Geometry: final body of the model. Coordinates: model frame, mm. A direction names the side the tool comes from. Round coordinates to 2 decimals unless told otherwise and drop trailing zeros. Loops run counter-clockwise (first coordinate to the right, second up) from the corner with the lowest first, then second, coordinate; pieces in that order, holes last. Notation, with made-up numbers: (33.5, 15.25) - (65.5, 15.25) arc R24 ccw to (65.5, 51.25) - close; hole circle Ø2 at (-26.5, 8.5). An arc over 180 degrees is marked (long way). Answer as a JSON object with one key per item and string values. Group by question number.
Item 1: Section A-A (z = 0). Return the cut outline in (x, y).
Item 2: Line query: line 1 (Z direction, x = -14, y = 2.2); line 2 (X direction, y = 1.25, z = 0); line 3 (X direction, y = 1.7, z = 16). Output: solid intervals per line, ascending.
Item 3: Section C-C (y = 0.65). Return the cut outline in (x, z).
Item 4: Section B-B (x = 1). Return the cut outline in (y, z), plus the area to 3 significant figures.
Item 5: Draft query along Z for faces 1 (the face through (-2, 1, -9)), 2 (the face through (2.863, 1.479, 0.969)), 3 (the face through (-9.248, 1.521, 9.713)). Return one class per face: released by +Z, released by -Z, zero draft, split by the parting line, or undercut.
Item 6: Reachability of faces 4 (the face through (-17.4, 1.48, 19.43)), 5 (the face through (-10, 1, -15)), 6 (the face through (-10, 1, 15)) from +Z, -Z, +X, -X, +Y, -Y: full face, straight path, thin tool, end or side. Return the list, or none.
Item 7: Section D-D (x = -14). Return the cut outline in (y, z), plus the area to 3 significant figures.
Item 8: First-contact query: pin 1 (0.9 mm diameter, centred on y = 1.5, z = 16, fed in from +X); pin 2 (4 mm diameter, centred on x = 1, z = 0, fed in from -Y). Flat tips, straight axial feed; report the tip coordinate or a pass-through.
Autodesk Inventor part; units mm, degrees
ref_plane "YZ Plane" through (0, 0, 0) normal (1, 0, 0) x (0, 1, 0)
ref_plane "XZ Plane" through (0, 0, 0) normal (0, 1, 0) x (-1, 0, 0)
ref_plane "XY Plane" through (0, 0, 0) normal (0, 0, 1) x (1, 0, 0)
sketch "スケッチ1" plane through (0, 0, 0) normal (0, 1, 0) x (-1, 0, 0)
  line L0 (-3, 9) -> (10, 9)
  line L1 (10, -9) -> (-3, -9)
  line L2 (-5, -7) -> (-5, 7)
  line L3 (12, 20) -> (16, 20)
  line L4 (18, 18) -> (18, -18)
  line L5 (16, -20) -> (12, -20)
  line L6 (10, -18) -> (10, -9)
  line L7 (10, 9) -> (10, 18)
  arc A0 (18, 18) -> (16, 20) centre (16, 18) ccw
  arc A1 (12, 20) -> (10, 18) centre (12, 18) ccw
  arc A2 (16, -20) -> (18, -18) centre (16, -18) ccw
  arc A3 (10, -18) -> (12, -20) centre (12, -18) ccw
  arc A4 (-5, -7) -> (-3, -9) centre (-3, -7) ccw
  arc A5 (-3, 9) -> (-5, 7) centre (-3, 7) ccw
  point P0 (0, 0)
  point P1 (-5, 9)
  point P2 (-5, -9)
  point P3 (10, 20)
  point P4 (18, -20)
  point P5 (18, 20)
  point P6 (10, -20)
  dimension "d0" = 5
  dimension "d2" = 8
  dimension "d3" = 8
  dimension "d4" = 18
  dimension "d5" = 9
  dimension "d6" = 40
  dimension "d7" = 20
  dimension "d8" = 10
  dimension "d10" = 2
extrude "プレート1" add sketch "スケッチ1" along normal blind 3
hole "穴1" at (-14, 3, 16) direction (0, -1, 0) diameter 4.2 end through all
hole "穴2" at (-14, 3, -16) direction (0, -1, 0) diameter 4.2 end through all
hole "穴3" at (1, 3, 0) direction (0, -1, 0) diameter 4.2 end through all
sketch "スケッチ2" plane through (0, 0, 0) normal (0, -1, 0) x (1, 0, 0)
  circle A0 centre (1, 0) radius 2.1
  circle A1 centre (-14, -16) radius 2.1
  circle A2 centre (-14, 16) radius 2.1
  line L0 (-10, 9) -> (3, 9)
  line L1 (-10, 18) -> (-10, 9)
  arc A3 (-10, 18) -> (-12, 20) centre (-12, 18) ccw
  line L2 (-16, 20) -> (-12, 20)
  arc A4 (-16, 20) -> (-18, 18) centre (-16, 18) ccw
  line L3 (-18, -18) -> (-18, 18)
  arc A5 (-18, -18) -> (-16, -20) centre (-16, -18) ccw
  line L4 (-12, -20) -> (-16, -20)
  arc A6 (-12, -20) -> (-10, -18) centre (-12, -18) ccw
  line L5 (-10, -9) -> (-10, -18)
  line L6 (3, -9) -> (-10, -9)
  arc A7 (3, -9) -> (5, -7) centre (3, -7) ccw
  line L7 (5, 7) -> (5, -7)
  arc A8 (5, 7) -> (3, 9) centre (3, 7) ccw
  point P0 (0, 0)
fillet "フィレット1" radius 2.5 2 edges at (-10, 1.5, 9) (-10, 1.5, -9)
equation "\"d3\" = d2"
equation "\"d18\" = Thickness"
equation "\"d28\" = Thickness"
equation "\"d37\" = Thickness"
equation "\"d9\" = Thickness"
equation "\"BendRadius\" = Thickness"
equation "\"BendReliefWidth\" = Thickness"
equation "\"BendReliefDepth\" = 0.5 * Thickness"
equation "\"CornerReliefSize\" = 4 * Thickness"
equation "\"MinimumRemnant\" = 2 * Thickness"
equation "\"TransitionRadius\" = BendRadius"
equation "\"JacobiRadiusSize\" = BendRadius"
equation "\"GapSize\" = Thickness"
properties part number "T_almite_braket"
Values:
{
 "1": {"outline": "(-18, 0) - (-1.1, 0) - (-1.1, 3) - (-18, 3) - close; (3.1, 0) - (5, 0) - (5, 3) - (3.1, 3) - close"},
 "2": {"line 1": "z = -20 to -18.1, -13.9 to 13.9, 18.1 to 20", "line 2": "x = -18 to -1.1, 3.1 to 5", "line 3": "x = -18 to -16.1, -11.9 to -10"},
 "3": {"outline": "(-18, -18) arc R2 ccw to (-16, -20) - (-12, -20) arc R2 ccw to (-10, -18) - (-10, -11.5) arc R2.5 cw to (-7.5, -9) - (3, -9) arc R2 ccw to (5, -7) - (5, 7) arc R2 ccw to (3, 9) - (-7.5, 9) arc R2.5 cw to (-10, 11.5) - (-10, 18) arc R2 ccw to (-12, 20) - (-16, 20) arc R2 ccw to (-18, 18) - close; hole circle Ø4.2 at (-14, -16); hole circle Ø4.2 at (-14, 16); hole circle Ø4.2 at (1, 0)"},
 "4": {"outline": "(0, -9) - (3, -9) - (3, -2.1) - (0, -2.1) - close; (0, 2.1) - (3, 2.1) - (3, 9) - (0, 9) - close", "area": "41.4 mm^2"},
 "5": {"face 1": "released by -Z", "face 2": "undercut", "face 3": "released by +Z"},
 "6": {"face 4": "+Z, -X, +Y, -Y", "face 5": "-Z, +X, +Y, -Y", "face 6": "+Z, +X, +Y, -Y"},
 "7": {"outline": "(0, -20) - (3, -20) - (3, -18.1) - (0, -18.1) - close; (0, -13.9) - (3, -13.9) - (3, 13.9) - (0, 13.9) - close; (0, 18.1) - (3, 18.1) - (3, 20) - (0, 20) - close", "area": "94.8 mm^2"},
 "8": {"pin 1": "stops at x = -10", "pin 2": "passes through"}
}
